from build123d import *

# Parameters (mm, degrees)
F0_W     = 25.4
F0_H     = 19.05
F1_DEPTH = 3.175
F3_DEPTH = 3.176


with BuildPart() as f1:
    # F0 (on Right) → F1 (new body)
    with BuildSketch(Plane.YZ):
        Rectangle(F0_W, F0_H)
    extrude(amount=-F1_DEPTH)

    # F2 (on face) → F3 (cut, through all)
    with BuildSketch(Plane.YZ):
        with BuildLine():
            ThreePointArc((-6.270625, -4.7625), (-8.255, -2.778125), (-10.239375, -4.7625))
            Line((-10.239375, -4.7625), (-6.270625, -4.7625))
        make_face()
        with BuildLine():
            ThreePointArc((10.239375, -4.7625), (8.255, -2.778125), (6.270625, -4.7625))
            Line((6.270625, -4.7625), (10.239375, -4.7625))
        make_face()
        with BuildLine():
            Line((10.239375, -4.7625), (6.270625, -4.7625))
            ThreePointArc((6.270625, -4.7625), (8.255, -6.746875), (10.239375, -4.7625))
        make_face()
        with BuildLine():
            Line((-6.270625, -4.7625), (-10.239375, -4.7625))
            ThreePointArc((-10.239375, -4.7625), (-8.255, -6.746875), (-6.270625, -4.7625))
        make_face()
    extrude(amount=-F3_DEPTH, mode=Mode.SUBTRACT)


solid = f1.part
Model file for the job. Use its own axes, mm. Give positions to 0.01 mm unless a question says otherwise; leave off trailing zeros. Loops run counter-clockwise (first coordinate to the right, second up) from the corner with the lowest first, then second, coordinate; pieces in that order, holes last.
1) Pull direction Z, two halves, no side cores. Call faces 1 (the flat face through (-2, 0, 9.525)), 2 (the flat face through (-2, 12.7, 0)), 3 (the cylindrical face through (-1.565, -10.088, -4.002)): +Z half, -Z half, draft (parallel to the pull), parting line (faces both ways), or undercut.
2) Wall check: line 1 (Y direction, x = -1.2, z = -6.5); line 2 (Y direction, x = -2.75, z = -6). Give the ranges that are in metal, low to high.
3) Saw through at B-B (z = -4.5). Write the cut outline in (x, y) (3 decimals).
4) Saw through at C-C (x = -1.65). Write the cut outline in (y, z) (1 decimal).
5) Saw through at A-A (y = 9.25). Write the cut outline in (x, z) (3 decimals), plus the area to 3 significant figures.
6) Saw through at D-D (y = -8.75). Write the cut outline in (x, z) (3 decimals).
Answer block:
1. face 1: +Z half
1. face 2: draft
1. face 3: undercut
2. line 1: y = -12.7 to -9.21, -7.3 to 7.3, 9.21 to 12.7
2. line 2: y = -12.7 to -9.81, -6.7 to 6.7, 9.81 to 12.7
3. outline: (-3.175, -12.7) - (0, -12.7) - (0, -10.222) - (-3.175, -10.222) - close; (-3.175, -6.288) - (0, -6.288) - (0, 6.288) - (-3.175, 6.288) - close; (-3.175, 10.222) - (0, 10.222) - (0, 12.7) - (-3.175, 12.7) - close
4. outline: (-12.7, -9.5) - (12.7, -9.5) - (12.7, 9.5) - (-12.7, 9.5) - close; hole circle Ø4 at (-8.3, -4.8); hole circle Ø4 at (8.3, -4.8)
5. outline: (-3.175, -9.525) - (0, -9.525) - (0, -6.479) - (-3.175, -6.479) - close; (-3.175, -3.046) - (0, -3.046) - (0, 9.525) - (-3.175, 9.525) - close
5. area: 49.6 mm2
6. outline: (-3.175, -9.525) - (0, -9.525) - (0, -6.684) - (-3.175, -6.684) - close; (-3.175, -2.841) - (0, -2.841) - (0, 9.525) - (-3.175, 9.525) - close
